Here's how the part is built. I have some questions about the finished solid (model axes, mm). Round coordinates to 2 decimals unless told otherwise and drop trailing zeros. Loops run counter-clockwise (first coordinate to the right, second up) from the corner with the lowest first, then second, coordinate; pieces in that order, holes last. Notation, with made-up numbers: (26.25, 10.5) -> (79.25, 10.5) arc R24 cw to (79.25, 29.5) -> close; hole circle Ø1 at (28, 28.25). An arc over 180 degrees is marked (long way). Use one line per item in the form item = value. Start each with the question number.
Item 1: Thinking about a two-plate mould opening in X: for faces 1 (the face through (-43.87, 12.79, 27.37)), 2 (the face through (6.776, 0.054, 52.972)), 3 (the face through (-45.161, 21.966, 24.555)), which applies, released by +X, released by -X, zero draft, split by the parting line, or undercut?
Item 2: If I drill on L1, parallel to Z at x = -8, y = 24.5; L2, parallel to Y at x = 0, z = 2.3 (3 decimals); L3, parallel to X at y = 8, z = 53.3 (3 decimals), over which ranges is the centre line in solid material (lowest first)? Write a range as [from, to].
Item 3: If we section it at D-D (y = 33.5): Write out the boundary of the cut face in (x, z).
Item 4: If we section it at B-B (x = 4): Write out the boundary of the cut face in (y, z).
Item 5: I'm going to push flat-ended pins straight in: pin 1 Ø3 at (x, y) = (-3.5, 25.5) entering from -Z; pin 2 Ø2 at (y, z) = (30.72, 24.5) entering from -X; pin 3 Ø3 at (y, z) = (20.72, 14.5) entering from +X; pin 4 Ø8 at (y, z) = (37.5, 5.5) entering from +X. Where does each tip first touch, or does it pass through?
Item 6: If we section it at A-A (z = 24.5): Write out the boundary of the cut face in (x, y), then the cut area to 3 significant figures.
Item 7: If we section it at C-C (x = -25): Write out the boundary of the cut face in (y, z).
```python
from build123d import *

# Parameters (mm, degrees)
SKETCH_1_R          = 5
SKETCH_1_R_2        = 1.225
SKETCH_1_R_3        = 1.025
EXTRUDE_1_DEPTH     = 55
SKETCH_2_W          = 57.132931415
SKETCH_2_H          = 47
CUT_EXTRUDE_1_DEPTH = 66
SKETCH_3_R          = 1.25
CUT_EXTRUDE_2_DEPTH = 49


with BuildPart() as part:
    # 스케치1 → 보스-돌출1 (new body)
    with BuildSketch(Plane.XY):
        with BuildLine():
            Line((11.674013781, 7.727703555), (-14, 46.512678751))
            Line((-14, 46.512678751), (-47.132931415, 46.512678751))
            Line((-47.132931415, 46.512678751), (-47.132931415, 14.921692086))
            Line((-47.132931415, 14.921692086), (-11, -8.660254038))
            ThreePointArc((-11, -8.660254038), (8.200906179, -11.346591463), (11.674013781, 7.727703555))
        make_face()
        Circle(SKETCH_1_R, mode=Mode.SUBTRACT)
        with Locations((0, 8)):
            Circle(SKETCH_1_R_2, mode=Mode.SUBTRACT)
        with Locations((0, 11)):
            Circle(SKETCH_1_R_2, mode=Mode.SUBTRACT)
        with Locations((7.778174593, 7.778174593)):
            Circle(SKETCH_1_R_2, mode=Mode.SUBTRACT)
        with Locations((8, 0)):
            Circle(SKETCH_1_R_2, mode=Mode.SUBTRACT)
        with Locations((11, 0)):
            Circle(SKETCH_1_R_2, mode=Mode.SUBTRACT)
        with Locations((7.778174593, -7.778174593)):
            Circle(SKETCH_1_R_2, mode=Mode.SUBTRACT)
        with Locations((0, -8)):
            Circle(SKETCH_1_R_2, mode=Mode.SUBTRACT)
        with Locations((0, -11)):
            Circle(SKETCH_1_R_2, mode=Mode.SUBTRACT)
        with Locations((-7.778174593, -7.778174593)):
            Circle(SKETCH_1_R_2, mode=Mode.SUBTRACT)
        with Locations((-8, 0)):
            Circle(SKETCH_1_R_3, mode=Mode.SUBTRACT)
        with Locations((-11, 0)):
            Circle(SKETCH_1_R_2, mode=Mode.SUBTRACT)
        with Locations((-7.778174593, 7.778174593)):
            Circle(SKETCH_1_R_2, mode=Mode.SUBTRACT)
    extrude(amount=EXTRUDE_1_DEPTH)

    # 스케치2 → 컷-돌출1 (cut)
    with BuildSketch(Plane(origin=(0, 46.512678751, 0), x_dir=(1, 0, 0), z_dir=(0, 1, 0))):
        with Locations((-14.566465708, -27.5)):
            Rectangle(SKETCH_2_W, SKETCH_2_H)
    extrude(amount=-CUT_EXTRUDE_1_DEPTH, mode=Mode.SUBTRACT)

    # 스케치3 → 컷-돌출2 (cut)
    with BuildSketch(Plane.ZY.offset(47.132931415)):
        with Locations(Location((24.5, 30.717185419, 0), (0, 0, 270))):
            Circle(SKETCH_3_R)
        with Locations(Location((14.5, 40.717185419, 0), (0, 0, 270))):
            Circle(SKETCH_3_R)
        with Locations(Location((34.5, 30.717185419, 0), (0, 0, 270))):
            Circle(SKETCH_3_R)
        with Locations(Location((24.5, 40.717185419, 0), (0, 0, 270))):
            Circle(SKETCH_3_R)
        with Locations(Location((14.5, 30.717185419, 0), (0, 0, 270))):
            Circle(SKETCH_3_R)
        with Locations(Location((34.5, 40.717185419, 0), (0, 0, 270))):
            Circle(SKETCH_3_R)
        with Locations(Location((14.5, 20.717185419, 0), (0, 0, 270))):
            Circle(SKETCH_3_R)
        with Locations(Location((24.5, 20.717185419, 0), (0, 0, 270))):
            Circle(SKETCH_3_R)
        with Locations(Location((34.5, 20.717185419, 0), (0, 0, 270))):
            Circle(SKETCH_3_R)
    extrude(amount=-CUT_EXTRUDE_2_DEPTH, mode=Mode.SUBTRACT)


solid = part.part
```
Values found:
q1.face_1 = released by -X
q1.face_2 = undercut
q1.face_3 = zero draft
q2.L1 = [0, 4], [51, 55]
q2.L2 = [-14, -12.225], [-9.775, -9.225], [-6.775, -5], [5, 6.775], [9.225, 9.775], [12.225, 25.363]
q2.L3 = [-36.527, -8.983], [-6.573, -1.225], [1.225, 6.573], [8.983, 11.494]
q3.outline = (-47.13, 0) -> (-5.39, 0) -> (-5.39, 4) -> (-43.13, 4) -> (-43.13, 51) -> (-5.39, 51) -> (-5.39, 55) -> (-47.13, 55) -> close
q4.outline = (-13.42, 0) -> (-3, 0) -> (-3, 4) -> (-13.42, 4) -> close; (-13.42, 51) -> (-3, 51) -> (-3, 55) -> (-13.42, 55) -> close; (3, 0) -> (19.32, 0) -> (19.32, 4) -> (3, 4) -> close; (3, 51) -> (19.32, 51) -> (19.32, 55) -> (3, 55) -> close
q5.pin_1 = 0
q5.pin_2 = through
q5.pin_3 = -43.13
q5.pin_4 = -5.58
q6.outline = (-47.13, 14.92) -> (-43.13, 12.31) -> (-43.13, 19.47) -> (-47.13, 19.47) -> close; (-47.13, 21.97) -> (-43.13, 21.97) -> (-43.13, 29.47) -> (-47.13, 29.47) -> close; (-47.13, 31.97) -> (-43.13, 31.97) -> (-43.13, 39.47) -> (-47.13, 39.47) -> close; (-47.13, 41.97) -> (-43.13, 41.97) -> (-43.13, 46.51) -> (-47.13, 46.51) -> close
q6.area = 102 mm2
q7.outline = (0.48, 0) -> (46.51, 0) -> (46.51, 4) -> (0.48, 4) -> close; (0.48, 51) -> (46.51, 51) -> (46.51, 55) -> (0.48, 55) -> close
